from build123d import *

# Parameters (mm, degrees)
SKETCH_3_R          = 1.621125
EXTRUDE_1_DEPTH     = 3.2
SKETCH_5_R          = 5.745
SKETCH_5_R_2        = 3.5
CUT_EXTRUDE_1_DEPTH = 0.64
CUT_EXTRUDE_1_DRAFT = -60
SKETCH_7_R          = 5.745
SKETCH_7_R_2        = 3.5
CUT_EXTRUDE_2_DEPTH = 0.64
CUT_EXTRUDE_2_DRAFT = -60


with BuildPart() as part:
    # 草图3 → 凸台-拉伸1 (new body)
    with BuildSketch(Plane.XY):
        Polygon((0, 4.041451884), (-3.5, 2.020725942), (-3.5, -2.020725942), (0, -4.041451884), (3.5, -2.020725942), (3.5, 2.020725942), align=None)
        Circle(SKETCH_3_R, mode=Mode.SUBTRACT)
    extrude(amount=-EXTRUDE_1_DEPTH)

    # 草图4 → 切除-旋转1 (revolve, cut)
    with BuildSketch(Plane(origin=(0, 0, 0), x_dir=(0, 0, -1), z_dir=(1, 0, 0)), mode=Mode.PRIVATE) as cut_revolve_1_sk:
        Polygon((0, 2.3), (0.391948664, 1.621125), (0.391948664, 0), (0, 0), align=None)
        Polygon((3.2, 0), (3.2, 2.3), (2.808051336, 1.621125), (2.808051336, 0), align=None)
    revolve(cut_revolve_1_sk.sketch.rotate(Axis((0, 0, 0), (0, 0, -1)), 90), axis=Axis((0, 0, 0), (0, 0, -1)), mode=Mode.SUBTRACT)


with BuildPart() as cut_extrude_1_tool:
    # 草图5 → 切除-拉伸1 (with draft: the straight prism first)
    with BuildSketch(Plane.XY):
        Circle(SKETCH_5_R)
        Circle(SKETCH_5_R_2, mode=Mode.SUBTRACT)
    extrude(amount=-CUT_EXTRUDE_1_DEPTH)
    # 切除-拉伸1: the draft: its side faces are tilted about the plane it starts from
    cut_extrude_1_sides = [cut_extrude_1_tool.faces().sort_by_distance(p)[0] for p in [
        (-5.745, 0, -0.32),
        (-3.5, 0, -0.32),
    ]]
    draft(cut_extrude_1_sides, Plane.XY, CUT_EXTRUDE_1_DRAFT)


with BuildPart() as part_1:
    add(part.part)

    # 切除-拉伸1: cut by cut_extrude_1_tool
    add(cut_extrude_1_tool.part, mode=Mode.SUBTRACT)


with BuildPart() as cut_extrude_2_tool:
    # 草图7 → 切除-拉伸2 (with draft: the straight prism first)
    with BuildSketch(Plane(origin=(0, 0, -3.2), x_dir=(-1, 0, 0), z_dir=(0, 0, -1))):
        Circle(SKETCH_7_R)
        Circle(SKETCH_7_R_2, mode=Mode.SUBTRACT)
    extrude(amount=-CUT_EXTRUDE_2_DEPTH)
    # 切除-拉伸2: the draft: its side faces are tilted about the plane it starts from
    cut_extrude_2_sides = [cut_extrude_2_tool.faces().sort_by_distance(p)[0] for p in [
        (5.745, 0, -2.88),
        (3.5, 0, -2.88),
    ]]
    draft(cut_extrude_2_sides, Plane(origin=(0, 0, -3.2), x_dir=(-1, 0, 0), z_dir=(0, 0, -1)), CUT_EXTRUDE_2_DRAFT)


with BuildPart() as part_2:
    add(part_1.part)

    # 切除-拉伸2: cut by cut_extrude_2_tool
    add(cut_extrude_2_tool.part, mode=Mode.SUBTRACT)


solid = part_2.part
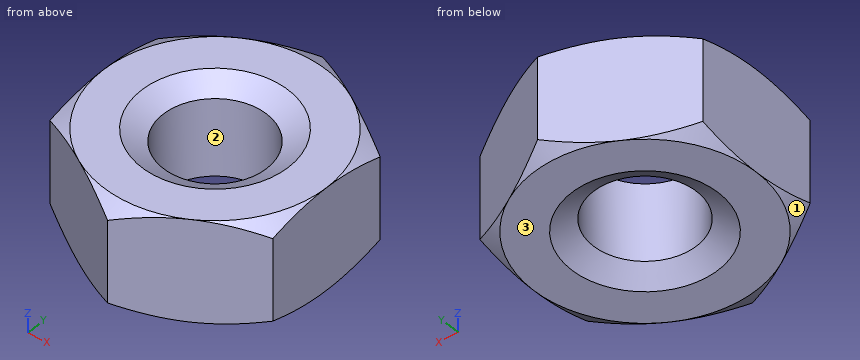
For this review, take the finished solid that the model builds, in its own axes (mm). Face numbers are marked on the shaded views. Round coordinates to 2 decimals unless told otherwise and drop trailing zeros. Write each loop counter-clockwise with the first axis right and the second up, starting at its lowest first coordinate (ties: lowest second). Pieces come first, ordered by that corner, then holes. Notation, with made-up numbers: (10.5, 41.5) - (28.5, 41.5) arc R28 cw to (28.5, 65.5) - close; hole circle Ø5 at (-34, 36). An arc over 180 degrees is marked (long way). Write item = value, one per line. Start each with the question number.
1. For pin 1 Ø3 at (x, y) = (-1.5, -2.5) entering from +Z, flat-tipped, find the tip position at first contact; note if it passes through.
2. Wall thickness on L1, parallel to Y at x = 1.25, z = -0.85; L2, parallel to Y at x = -1, z = -2.15; L3, parallel to Y at x = 2.25, z = -1.85: over which ranges is each line inside the solid? List them lowest first.
3. Consider section A-A on z = -1.8. State the section outline as (x, y) points.
4. Draft analysis for pull direction Y (two halves, no side actions). For the marked faces 1, 2 and 3, state which applies: released by +Y, released by -Y, zero draft, split by the parting line, or undercut.
Evaluation:
q1.pin_1 = 0
q2.L1 = -3.32 to -1.03, 1.03 to 3.32
q2.L2 = -3.46 to -1.28, 1.28 to 3.46
q2.L3 = -2.74 to 2.74
q3.outline = (-3.5, -2.02) - (0, -4.04) - (3.5, -2.02) - (3.5, 2.02) - (0, 4.04) - (-3.5, 2.02) - close; hole circle Ø3.24 at (0, 0)
q4.face_1 = released by -Y
q4.face_2 = undercut
q4.face_3 = zero draft
